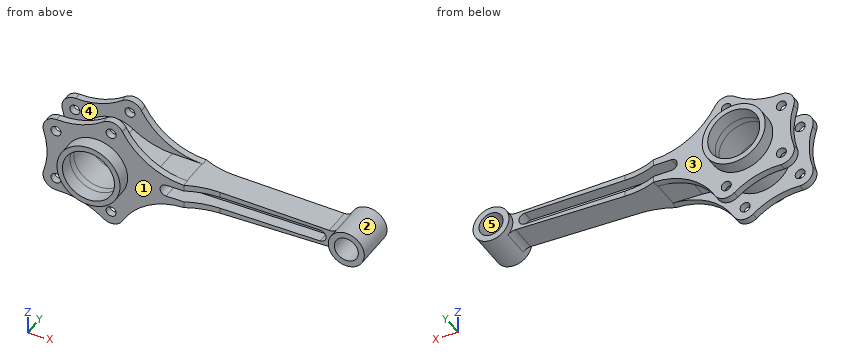
from build123d import *

# Parameters (mm, degrees)
SKETCH1_R           = 31.5
SKETCH1_R_2         = 26
BOSS_EXTRUDE1_DEPTH = 35
SKETCH1_3_R         = 18
SKETCH1_3_R_2       = 12
BOSS_EXTRUDE2_DEPTH = 21
BOSS_EXTRUDE3_DEPTH = 17.5
BOSS_EXTRUDE4_DEPTH = 14
SKETCH3_R           = 5
BOSS_EXTRUDE5_DEPTH = 7
BOSS_EXTRUDE6_REACH = 58
BOSS_EXTRUDE9_REACH = 58
SKETCH6_R           = 26
CUT_EXTRUDE1_DEPTH  = 42
CUT_EXTRUDE2_DEPTH  = 23


with BuildPart() as part:
    # Sketch1 → Boss-Extrude1 (new body, symmetric)
    with BuildSketch(Plane(origin=(0, 0, 0), x_dir=(1, 0, 0), z_dir=(0, 1, 0))):
        Circle(SKETCH1_R)
        Circle(SKETCH1_R_2, mode=Mode.SUBTRACT)
    extrude(amount=BOSS_EXTRUDE1_DEPTH, both=True)

    # Sketch1<5> → Boss-Extrude3 (add, symmetric)
    with BuildSketch(Plane(origin=(0, 0, 0), x_dir=(1, 0, 0), z_dir=(0, 1, 0))):
        with BuildLine():
            ThreePointArc((17.981178031, -25.863627677), (36.746938107, -16.532049941), (57.405028955, -13))
            Line((57.405028955, -13), (87, -12.310914466))
            Line((87, -12.310914466), (87, 12.310914466))
            Line((87, 12.310914466), (57.405028955, 13))
            ThreePointArc((57.405028955, 13), (36.746938107, 16.532049941), (17.981178031, 25.863627677))
            ThreePointArc((17.981178031, 25.863627677), (27.916456688, 14.591828056), (31.5, 0))
            ThreePointArc((31.5, 0), (27.916456688, -14.591828056), (17.981178031, -25.863627677))
        make_face()
    extrude(amount=BOSS_EXTRUDE3_DEPTH, both=True)



with BuildPart() as body_2:
    # Sketch1<3> → Boss-Extrude2 (new body, symmetric)
    with BuildSketch(Plane(origin=(0, 0, 0), x_dir=(1, 0, 0), z_dir=(0, 1, 0))):
        with Locations((250, 0)):
            Circle(SKETCH1_3_R)
        with Locations((250, 0)):
            Circle(SKETCH1_3_R_2, mode=Mode.SUBTRACT)
    extrude(amount=BOSS_EXTRUDE2_DEPTH, both=True)


with BuildPart() as part_1:
    add(part.part)

    add(body_2.part)  # Boss-Extrude4 merges body 2
    # Sketch1<6> → Boss-Extrude4 (add, symmetric)
    with BuildSketch(Plane(origin=(0, 0, 0), x_dir=(1, 0, 0), z_dir=(0, 1, 0))):
        with BuildLine():
            Line((87, 12.310914466), (87, -12.310914466))
            Line((87, -12.310914466), (229.197757742, -9))
            ThreePointArc((229.197757742, -9), (233.333153837, -9.790252147), (236.776771457, -12.212543834))
            ThreePointArc((236.776771457, -12.212543834), (232, 0), (236.776771457, 12.212543834))
            ThreePointArc((236.776771457, 12.212543834), (233.333153837, 9.790252147), (229.197757742, 9))
            Line((229.197757742, 9), (87, 12.310914466))
        make_face()
    extrude(amount=BOSS_EXTRUDE4_DEPTH, both=True)

    # Sketch3 → Boss-Extrude5 (add)
    with BuildSketch(Plane(origin=(0, 14, 0), x_dir=(1, 0, 0), z_dir=(0, 1, 0))):
        with BuildLine():
            Line((87.628988844, 12.29626917), (87.628988844, -12.29626917))
            ThreePointArc((87.628988844, -12.29626917), (52.070762211, -22.651980063), (26.364290052, -49.312916252))
            ThreePointArc((26.364290052, -49.312916252), (17.700433018, -55.716432735), (7.181946677, -53.386435492))
            ThreePointArc((7.181946677, -53.386435492), (-14.855989459, -42.122318837), (-39.406288617, -38.986435492))
            ThreePointArc((-39.406288617, -38.986435492), (-50.326951915, -33.896458963), (-52.376901133, -22.023529412))
            ThreePointArc((-52.376901133, -22.023529412), (-48.925892025, 0), (-52.376901133, 22.023529412))
            ThreePointArc((-52.376901133, 22.023529412), (-50.326951915, 33.896458963), (-39.406288617, 38.986435492))
            ThreePointArc((-39.406288617, 38.986435492), (-14.855989459, 42.122318837), (7.181946677, 53.386435492))
            ThreePointArc((7.181946677, 53.386435492), (17.700433018, 55.716432735), (26.364290052, 49.312916252))
            ThreePointArc((26.364290052, 49.312916252), (52.070762211, 22.651980063), (87.628988844, 12.29626917))
        make_face()
        with Locations((15, 43)):
            Circle(SKETCH3_R, mode=Mode.SUBTRACT)
        with Locations((-40, 26)):
            Circle(SKETCH3_R, mode=Mode.SUBTRACT)
        with Locations((-40, -26)):
            Circle(SKETCH3_R, mode=Mode.SUBTRACT)
        with Locations((15, -43)):
            Circle(SKETCH3_R, mode=Mode.SUBTRACT)
    boss_extrude5 = extrude(amount=BOSS_EXTRUDE5_DEPTH)

    # Mirror1: Boss-Extrude5 across plane
    add(boss_extrude5.mirror(Plane.ZX))

    # Boss-Extrude6: up to this face of the body (flat: up to its plane)
    boss_extrude6_end = Plane(part_1.part.faces().sort_by_distance((143.301393348, 0, 11))[0])
    # Sketch4 → Boss-Extrude6 (add, up to the picked face)
    with BuildSketch(Plane.XY, mode=Mode.PRIVATE) as boss_extrude6_sk1:
        with BuildLine():
            Line((87.628988844, 21), (87.628988844, 14))
            Line((87.628988844, 14), (119.924499368, 14))
            ThreePointArc((119.924499368, 14), (103.401787726, 15.770084612), (87.628988844, 21))
        make_face()
    boss_extrude6_tool1 = split(extrude(boss_extrude6_sk1.sketch, amount=BOSS_EXTRUDE6_REACH, mode=Mode.PRIVATE), bisect_by=boss_extrude6_end, keep=Keep.BOTH, mode=Mode.PRIVATE)
    add(boss_extrude6_tool1.solids().sort_by_distance((95.628627, 16.082796, 0))[0])
    # Sketch4 → Boss-Extrude6 (add, up to the picked face)
    with BuildSketch(Plane.XY, mode=Mode.PRIVATE) as boss_extrude6_sk2:
        with BuildLine():
            Line((87.628988844, -21), (87.628988844, -14))
            Line((87.628988844, -14), (119.924499368, -14))
            ThreePointArc((119.924499368, -14), (103.401787726, -15.770084612), (87.628988844, -21))
        make_face()
    boss_extrude6_tool2 = split(extrude(boss_extrude6_sk2.sketch, amount=BOSS_EXTRUDE6_REACH, mode=Mode.PRIVATE), bisect_by=boss_extrude6_end, keep=Keep.BOTH, mode=Mode.PRIVATE)
    add(boss_extrude6_tool2.solids().sort_by_distance((95.628627, -16.082796, 0))[0])

    # Boss-Extrude9: up to this face of the body (flat: up to its plane)
    boss_extrude9_end = Plane(part_1.part.faces().sort_by_distance((143.301393348, 0, -11))[0])
    # Sketch5 → Boss-Extrude9 (add, up to the picked face)
    with BuildSketch(Plane(origin=(0, 0, 0), x_dir=(-1, 0, 0), z_dir=(0, 0, -1)), mode=Mode.PRIVATE) as boss_extrude9_sk1:
        with BuildLine():
            Line((-119.924499368, -14), (-87.628988844, -14))
            Line((-87.628988844, -14), (-87.628988844, -21))
            ThreePointArc((-87.628988844, -21), (-103.401787726, -15.770084612), (-119.924499368, -14))
        make_face()
    boss_extrude9_tool1 = split(extrude(boss_extrude9_sk1.sketch, amount=BOSS_EXTRUDE9_REACH, mode=Mode.PRIVATE), bisect_by=boss_extrude9_end, keep=Keep.BOTH, mode=Mode.PRIVATE)
    add(boss_extrude9_tool1.solids().sort_by_distance((95.628627, -16.082796, 0))[0])
    # Sketch5 → Boss-Extrude9 (add, up to the picked face)
    with BuildSketch(Plane(origin=(0, 0, 0), x_dir=(-1, 0, 0), z_dir=(0, 0, -1)), mode=Mode.PRIVATE) as boss_extrude9_sk2:
        with BuildLine():
            Line((-119.924499368, 14), (-87.628988844, 14))
            Line((-87.628988844, 14), (-87.628988844, 21))
            ThreePointArc((-87.628988844, 21), (-103.401787726, 15.770084612), (-119.924499368, 14))
        make_face()
    boss_extrude9_tool2 = split(extrude(boss_extrude9_sk2.sketch, amount=BOSS_EXTRUDE9_REACH, mode=Mode.PRIVATE), bisect_by=boss_extrude9_end, keep=Keep.BOTH, mode=Mode.PRIVATE)
    add(boss_extrude9_tool2.solids().sort_by_distance((95.628627, 16.082796, 0))[0])

    # Sketch6 → Cut-Extrude1 (cut)
    with BuildSketch(Plane(origin=(0, 21, 0), x_dir=(1, 0, 0), z_dir=(0, 1, 0))):
        Circle(SKETCH6_R)
    extrude(amount=-CUT_EXTRUDE1_DEPTH, mode=Mode.SUBTRACT)

    # Sketch7 → Cut-Extrude2 (cut)
    with BuildSketch(Plane(origin=(0, 2.5, 0), x_dir=(1, 0, 0), z_dir=(0, 1, 0))):
        with BuildLine():
            Line((220, -6), (70, -6))
            ThreePointArc((70, -6), (64, 0), (70, 6))
            Line((70, 6), (220, 6))
            ThreePointArc((220, 6), (226, 0), (220, -6))
        make_face()
    cut_extrude2 = extrude(amount=CUT_EXTRUDE2_DEPTH, mode=Mode.SUBTRACT)

    # Mirror2: Cut-Extrude2 across plane
    add(cut_extrude2.mirror(Plane.ZX), mode=Mode.SUBTRACT)


solid = part_1.part
Check sheet for the modelled part. Datum: model origin and axes. Units: mm. Face numbers are marked on the shaded views. A direction names the side the tool comes from. Round coordinates to 2 decimals unless told otherwise and drop trailing zeros. Loops run counter-clockwise (first coordinate to the right, second up) from the corner with the lowest first, then second, coordinate; pieces in that order, holes last.
1. Mould release check, pull along X, two halves, no side actions. Record for the marked faces 1 and 2: released by +X, released by -X, zero draft, split by the parting line, or undercut.
2. Sectioned sample at B-B on z = 43. Record the boundary of the cut face in (x, y), and give its area (3 significant figures).
3. Sectioned sample at A-A on x = 250. Record the boundary of the cut face in (y, z).
4. Sectioned sample at C-C on x = 124.5. Record the boundary of the cut face in (y, z).
5. Sectioned sample at D-D on y = -26. Record the boundary of the cut face in (x, z).
6. Scan lines: probe 1 along Z at (x, y) = (-40, 16.25); probe 2 along X at (y, z) = (29, 0); probe 3 along X at (y, z) = (-14.5, -4). Record each from-to range of solid material in increasing order.
7. Gauge pin test, flat ends, axial feed: pin 1 Ø2 at (x, y) = (14, -6.5) entering from -Z; pin 2 Ø21.5 at (x, z) = (250, 0) entering from -Y; pin 3 Ø7.5 at (x, z) = (188, -0.5) entering from +Y; pin 4 Ø16 at (x, z) = (-40, -26) entering from -Y. Record the tip position at first contact, or that the pin passes through.
8. Set-up check for the marked faces 3, 4 and 5: record each of +Z, -Z, +X, -X, +Y, -Y from which the full face is reachable in a straight line by a thin tool's end or side.
Recorded:
1. face 1: zero draft
1. face 2: undercut
2. outline: (-12.2, -21) - (10, -21) - (10, -14) - (-12.2, -14) - close; (-12.2, 14) - (10, 14) - (10, 21) - (-12.2, 21) - close; (20, -21) - (30.31, -21) - (30.31, -14) - (20, -14) - close; (20, 14) - (30.31, 14) - (30.31, 21) - (20, 21) - close
2. area: 455 mm2
3. outline: (-21, -18) - (21, -18) - (21, -12) - (-21, -12) - close; (-21, 12) - (21, 12) - (21, 18) - (-21, 18) - close
4. outline: (-14, -11.44) - (14, -11.44) - (14, -6) - (2.5, -6) - (2.5, 6) - (14, 6) - (14, 11.44) - (-14, 11.44) - (-14, 6) - (-2.5, 6) - (-2.5, -6) - (-14, -6) - close
5. outline: circle Ø63 at (0, 0); hole circle Ø52 at (0, 0)
6. probe 1: z = -39 to -31, -21 to 21, 31 to 39
6. probe 2: x = -31.5 to -26, 26 to 31.5
6. probe 3: x = -49.04 to -25.69, 25.69 to 65.53, 232.45 to 238.69, 261.31 to 267.55
7. pin 1: stops at z = -28.69
7. pin 2: passes through
7. pin 3: stops at y = 2.5
7. pin 4: stops at y = -21
8. face 3: +Y
8. face 4: none
8. face 5: +Y, -Y
